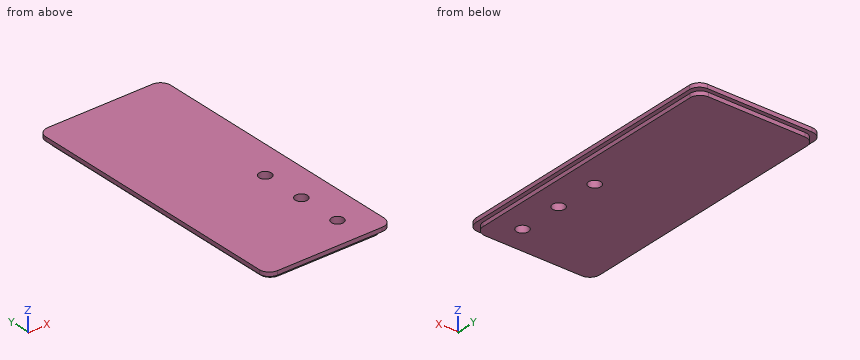
Solid Edge part; units mm, degrees
sketch "Sketch1" plane through (0, 0, 0) normal (0, 0, 1) x (1, 0, 0)
  line L0 (-31, -70) -> (31, -70)
  line L1 (31, -70) -> (31, 70)
  line L2 (31, 70) -> (-31, 70)
  line L3 (-31, 70) -> (-31, -70)
  dimension "D1" = 31
  dimension "D2" = 31
extrude "Ajout_matière_1" add sketch "Sketch1" along normal blind 2
fillet "Congé_1" radius 5 4 edges at (-31, -70, 1) (31, -70, 1) (-31, 70, 1) (31, 70, 1)
sketch "Sketch2" plane through (0, 0, 0) normal (0, 0, -1) x (-1, 0, 0)
  line L0 (-29, -68) -> (29, -68)
  line L1 (29, -68) -> (29, 68)
  line L2 (29, 68) -> (-29, 68)
  line L3 (-29, 68) -> (-29, -68)
extrude "Ajout_matière_2" add sketch "Sketch2" along normal blind 2
fillet "Congé_2" radius 5 4 edges at (29, 68, -1) (-29, 68, -1) (-29, -68, -1) (29, -68, -1)
hole "Perçage_1" at (16, -55, 2) direction (0, 0, -1) diameter 6 end up to next
hole "Hole1" at (16, -33, 2) direction (0, 0, -1) diameter 6 end up to next
hole "Hole2" at (16, -11, 2) direction (0, 0, -1) diameter 6 end up to next
properties material "Acier S235"
Build history of the part. All positions in model axes, mm. Round coordinates to 2 decimals unless told otherwise and drop trailing zeros. Order: outer loops, then holes, each group sorted by start corner. A loop starts at its lowest first (then second) coordinate and runs counter-clockwise, first axis right, second up. Notation, with made-up numbers: M 68,-22 L 107,-22 A31 ccw 107,7 Z; hole C -7,-5 d9. An arc over 180 degrees is marked long. Use CSV: the item, a comma, the result in double quotes. Start each with the question number.
(1) Cut at D-D on y = 28.5. List the corners of the cut face in (x, z), then the cut area to 3 significant figures.
(2) Drill centre lines: probe 1 along Y at (x, z) = (16, 1.15); probe 2 along Y at (x, z) = (16, -0.85); probe 3 along X at (y, z) = (-33, -0.3). Where is each one in solid material? Low to high.
(3) Flat gauge pins, fed straight in: P1, Ø2, axis at y = -16.5, z = -1.5, coming from the +X side; P2, Ø0.6, axis at x = 4, z = -1, coming from the +Y side; P3, Ø1.6, axis at y = -19, z = -1, coming from the -X side; P4, Ø3.5, axis at x = 16, y = -55, coming from the -Z side. Where does each tip first touch, or does it go through?
(4) Cut at B-B on z = -1. List the corners of the cut face in (x, y), then the cut area to 3 significant figures.
(5) Cut at C-C on y = -55. List the corners of the cut face in (x, z).
(6) Cut at A-A on x = 16. List the corners of the cut face in (y, z).
Findings:
1,outline,"M -31,0 L -29,0 L -29,-2 L 29,-2 L 29,0 L 31,0 L 31,2 L -31,2 Z"
1,area,"240 mm^2"
2,probe 1,"y = -70 to -58, -52 to -36, -30 to -14, -8 to 70"
2,probe 2,"y = -68 to -58, -52 to -36, -30 to -14, -8 to 68"
2,probe 3,"x = -29 to 13, 19 to 29"
3,P1,"stops at x = 29"
3,P2,"stops at y = 68"
3,P3,"stops at x = -29"
3,P4,"passes through"
4,outline,"M -29,-63 A5 ccw -24,-68 L 24,-68 A5 ccw 29,-63 L 29,63 A5 ccw 24,68 L -24,68 A5 ccw -29,63 Z; hole C 16,-55 d6; hole C 16,-33 d6; hole C 16,-11 d6"
4,area,"7,780 mm^2"
5,outline,"M -31,0 L -29,0 L -29,-2 L 13,-2 L 13,2 L -31,2 Z; M 19,-2 L 29,-2 L 29,0 L 31,0 L 31,2 L 19,2 Z"
6,outline,"M -70,0 L -68,0 L -68,-2 L -58,-2 L -58,2 L -70,2 Z; M -52,-2 L -36,-2 L -36,2 L -52,2 Z; M -30,-2 L -14,-2 L -14,2 L -30,2 Z; M -8,-2 L 68,-2 L 68,0 L 70,0 L 70,2 L -8,2 Z"
